Work out the finished part from the listing and answer in its coordinate system (mm). A direction names the side the tool comes from. Give positions to 0.01 mm unless a question says otherwise; leave off trailing zeros. Write each loop counter-clockwise with the first axis right and the second up, starting at its lowest first coordinate (ties: lowest second). Pieces come first, ordered by that corner, then holes.
1) Find section A-A (z = 9). Determine the outline of the cut face in (x, y), plus the area to 3 significant figures.
2) A tool of negligible diameter and unlimited length cuts with its end or side. For faces 5 (the face through (-8.493, -19.433, 24.605)), 6 (the face through (-1.5, -11, 14.8)), from which of +Z, -Z, +X, -X, +Y, -Y can it reach the whole face along a straight path? Write none if from no direction.
3) Find section B-B (y = -2). Determine the outline of the cut face in (x, z), plus the area to 3 significant figures.
4) Straight lines are drawn through the part: probe 1 along X at (y, z) = (-21.25, 24.5); probe 2 along Y at (x, z) = (-2, 1.5); probe 3 along Z at (x, y) = (-18.5, -4). For each, find the intervals that lie inside material, in ascending order.
5) Determine the mould class of faces 1 (the face through (0, -5, 15)), 2 (the face through (-12.08, -9.55, 22.74)), 3 (the face through (-1.642, -23.651, 28.722)), 4 (the face through (-10, -12, 0)) for opening direction X: pulls with the +X half, pulls with the -X half, needs draft (parallel to the pull), parting line crosses it, or undercut.
6) Given pin 1 Ø12 at (y, z) = (-8, 25.5) entering from +X; pin 2 Ø4 at (x, y) = (-9.5, -11) entering from +Z; pin 3 Ø1.5 at (x, y) = (-16.5, -11.5) entering from +Z, each flat-ended and moving along its own axis, determine where each tip first touches the part or whether it passes through.
```python
from build123d import *

# Parameters (mm, degrees)
F1_DEPTH = 25
F3_DEPTH = 30.001
F6_R     = 0.25
F7_DEPTH = 41.0214813745


with BuildPart() as f1:
    # F0 (on Front) → F1 (new body)
    with BuildSketch(Plane.XZ):
        Polygon((-20, 0), (0, 0), (0, 30), (-20, 17.9827876194), align=None)
    extrude(amount=F1_DEPTH)

    # F2 (on face) → F3 (cut, through all)
    with BuildSketch(Plane(origin=(0, 0, 0), x_dir=(1, 0, 0), z_dir=(0, 0, -1))):
        Polygon((0, 9.5), (0, 15.5), (-3, 12.5), align=None)
    extrude(amount=-F3_DEPTH, mode=Mode.SUBTRACT)

    # F6 (on line) → F7 (cut, through all)
    with BuildSketch(Plane(origin=(9.0046896383, 7.208208517, 5.4105633902), x_dir=(-0.4849657456, 0.8245581362, -0.2913968181), z_dir=(0.7067842719, 0.5657772353, 0.4246788351))):
        with Locations((-17.0687173915, 25.7150190211)):
            Circle(F6_R)
        with Locations((-19.0687173915, 25.7150190211)):
            Circle(F6_R)
        with Locations((-21.0687173915, 25.7150190211)):
            Circle(F6_R)
        with Locations((-23.0687173915, 25.7150190211)):
            Circle(F6_R)
        with Locations((-25.0687173915, 25.7150190211)):
            Circle(F6_R)
        with Locations((-27.0687173915, 25.7150190211)):
            Circle(F6_R)
    extrude(amount=-F7_DEPTH, mode=Mode.SUBTRACT)


solid = f1.part
```
Results:
1. outline: (-20, -25) - (0, -25) - (0, -15.5) - (-3, -12.5) - (0, -9.5) - (0, 0) - (-20, 0) - close
1. area: 491 mm2
2. face 5: none
2. face 6: +Z, -Z, +X
3. outline: (-20, 0) - (0, 0) - (0, 30) - (-20, 17.98) - close
3. area: 480 mm2
4. probe 1: x = -9.15 to 0
4. probe 2: y = -25 to -13.5, -11.5 to 0
4. probe 3: z = 0 to 18.88
5. face 1: pulls with the +X half
5. face 2: pulls with the -X half
5. face 3: undercut
5. face 4: needs draft
6. pin 1: stops at x = 0
6. pin 2: stops at z = 25.49
6. pin 3: stops at z = 20.54
